```python
from build123d import *

# Parameters (mm, degrees)
SKETCH1_W                     = 289.56
SKETCH1_H                     = 289.56
BOSS_EXTRUDE1_DEPTH           = 12.7
PIPE_TAP_DRILL_FOR_1_4_TAP2_D = 11.1252
PIPE_TAP_DRILL_FOR_1_4_TAP1_D = 11.1252
F_1_4_CLEARANCE_HOLE1_D       = 6.7564
SKETCH12_R                    = 127.635
SKETCH12_R_2                  = 123.19
CUT_EXTRUDE1_DEPTH            = 9.525
CIRPATTERN1_COUNT             = 4


with BuildPart() as part:
    # Sketch1 → Boss-Extrude1 (new body)
    with BuildSketch(Plane(origin=(0, 0, 0), x_dir=(1, 0, 0), z_dir=(0, 1, 0))):
        Rectangle(SKETCH1_W, SKETCH1_H)
    extrude(amount=BOSS_EXTRUDE1_DEPTH)

    # Pipe Tap Drill for 1/4 Tap2 (through all)
    with Locations(Plane(origin=(0, 12.7, 0), x_dir=(1, 0, 0), z_dir=(0, 1, 0))):
        with Locations((0, 0)):
            Hole(PIPE_TAP_DRILL_FOR_1_4_TAP2_D / 2)

    # Pipe Tap Drill for 1/4 Tap1 (through all)
    with Locations(Plane(origin=(0, 12.7, 0), x_dir=(1, 0, 0), z_dir=(0, 1, 0))):
        with Locations((-40.411152545, -40.411152545)):
            Hole(PIPE_TAP_DRILL_FOR_1_4_TAP1_D / 2)

    # 1/4 Clearance Hole1 (through all)
    with Locations(Plane(origin=(0, 12.7, 0), x_dir=(1, 0, 0), z_dir=(0, 1, 0))):
        with Locations((-98.782817332, -98.782817332)):
            f_1_4_clearance_hole1 = Hole(F_1_4_CLEARANCE_HOLE1_D / 2)

    # Sketch12 → Cut-Extrude1 (cut)
    with BuildSketch(Plane.XZ):
        Circle(SKETCH12_R)
        Circle(SKETCH12_R_2, mode=Mode.SUBTRACT)
    extrude(amount=-CUT_EXTRUDE1_DEPTH, mode=Mode.SUBTRACT)

    # CirPattern1: 1/4 Clearance Hole1 ×4 about axis
    cirpattern1_axis = Axis((0, 0, 0), (0, 1, 0))
    for i in range(1, CIRPATTERN1_COUNT):
        add(f_1_4_clearance_hole1.rotate(cirpattern1_axis, i * 360 / CIRPATTERN1_COUNT), mode=Mode.SUBTRACT)


solid = part.part
```
Geometry check sheet. Reference: the model listing, model coordinates, mm. A direction names the side the tool comes from. Give positions to 0.01 mm unless a question says otherwise; leave off trailing zeros. Order: outer loops, then holes, each group sorted by start corner. A loop starts at its lowest first (then second) coordinate and runs counter-clockwise, first axis right, second up. Notation, with made-up numbers: (27.5, 83) -> (78.5, 83) arc R14 ccw to (78.5, 93) -> close; hole circle Ø5 at (82.25, -14.75). An arc over 180 degrees is marked (long way). Write each question's results on one line, items separated by ' | '. Start each with the question number.
(1) Mould release check, pull along Z, two halves, no side actions. Record for faces 1 (the face through (98.63, 6.26, 95.41)), 2 (the face through (-2, 6, 144.78)), 3 (the face through (-2, 6, -144.78)): pulls with the +Z half, pulls with the -Z half, needs draft (parallel to the pull), parting line crosses it, or undercut.
(2) Sectioned sample at A-A (x = 0). Enter the section's corners in (y, z) (3 decimals), plus the area to 3 significant figures.
(3) Sectioned sample at D-D (z = -87). Enter the section's corners in (x, y) (3 decimals), plus the area to 3 significant figures.
(4) Scan lines: line 1 (Z direction, x = 0, y = 4.5) (3 decimals); line 2 (Z direction, x = -41.5, y = 7.5); line 3 (X direction, y = 9, z = -11.5). Record each from-to range of solid material in increasing order.
(5) Sectioned sample at B-B (z = 0). Enter the section's corners in (x, y) (3 decimals).
(6) Sectioned sample at C-C (y = 3.75). Give the number of separate pieces and of enclosed holes in the cut face, plus the area to 3 significant figures.
(7) Access from +Z, -Z, +X, -X, +Y, -Y to the whole of each face (thin tool, end or side, straight path). Record for faces 4 (the face through (-5.306, 6.261, -1.671)), 5 (the face through (-67, 9.525, 105)).
Answer below:
1) face 1: undercut | face 2: pulls with the +Z half | face 3: pulls with the -Z half
2) outline: (0, -144.78) -> (12.7, -144.78) -> (12.7, -5.563) -> (0, -5.563) -> (0, -123.19) -> (9.525, -123.19) -> (9.525, -127.635) -> (0, -127.635) -> close; (0, 5.563) -> (12.7, 5.563) -> (12.7, 144.78) -> (0, 144.78) -> (0, 127.635) -> (9.525, 127.635) -> (9.525, 123.19) -> (0, 123.19) -> close | area: 3,450 mm2
3) outline: (-144.78, 0) -> (-93.39, 0) -> (-93.39, 9.525) -> (-87.217, 9.525) -> (-87.217, 0) -> (87.217, 0) -> (87.217, 9.525) -> (93.39, 9.525) -> (93.39, 0) -> (144.78, 0) -> (144.78, 12.7) -> (-144.78, 12.7) -> close | area: 3,560 mm2
4) line 1: -144.78 to -127.635, -123.19 to -5.563, 5.563 to 123.19, 127.635 to 144.78 | line 2: -144.78 to -120.7, -115.99 to 34.96, 45.87 to 115.99, 120.7 to 144.78 | line 3: -144.78 to -127.12, -122.65 to 122.65, 127.12 to 144.78
5) outline: (-144.78, 0) -> (-127.635, 0) -> (-127.635, 9.525) -> (-123.19, 9.525) -> (-123.19, 0) -> (-5.563, 0) -> (-5.563, 12.7) -> (-144.78, 12.7) -> close; (5.563, 0) -> (123.19, 0) -> (123.19, 9.525) -> (127.635, 9.525) -> (127.635, 0) -> (144.78, 0) -> (144.78, 12.7) -> (5.563, 12.7) -> close
6) separate pieces: 2 | enclosed holes: 7 | area: 80,000 mm2
7) face 4: +Y, -Y | face 5: -Y
